```python
from build123d import *

# Parameters (mm, degrees)
SKETCH1_W           = 106.68
SKETCH1_H           = 38.1
BOSS_EXTRUDE1_DEPTH = 12.7
SKETCH2_R           = 3.2639
CUT_EXTRUDE1_DEPTH  = 22.225
CUT_EXTRUDE2_START  = -22.225
SKETCH3_R           = 3.2639
CUT_EXTRUDE2_DEPTH  = 22.225


with BuildPart() as part:
    # Sketch1 → Boss-Extrude1 (new body)
    with BuildSketch(Plane.XY):
        Rectangle(SKETCH1_W, SKETCH1_H)
    extrude(amount=BOSS_EXTRUDE1_DEPTH)

    # Sketch2 → Cut-Extrude1 (cut)
    with BuildSketch(Plane(origin=(53.34, 0, 0), x_dir=(0, 0, -1), z_dir=(1, 0, 0))):
        with Locations((-6.35, 10.16)):
            Circle(SKETCH2_R)
        with Locations(Location((-6.35, -10.16, 0), (0, 0, 180))):
            Circle(SKETCH2_R)
    extrude(amount=-CUT_EXTRUDE1_DEPTH, mode=Mode.SUBTRACT)

    # Sketch3 → Cut-Extrude2 (cut)
    with BuildSketch(Plane.ZY.offset(53.34).offset(CUT_EXTRUDE2_START)):
        with Locations(Location((6.35, 10.16, 0), (0, 0, 180))):
            Circle(SKETCH3_R)
        with Locations((6.35, -10.16)):
            Circle(SKETCH3_R)
    extrude(amount=CUT_EXTRUDE2_DEPTH, mode=Mode.SUBTRACT)


solid = part.part
```
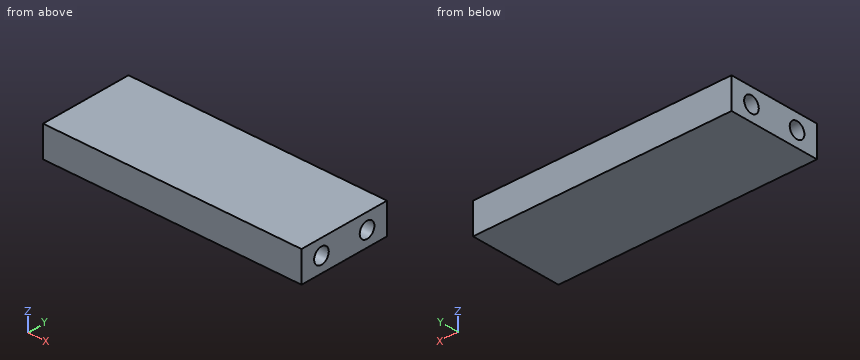
Could you check a few things on this model? Use its own coordinates, in mm. Coordinates: 2 decimals unless noted, no trailing zeros. Write each loop counter-clockwise with the first axis right and the second up, starting at its lowest first coordinate (ties: lowest second). Pieces come first, ordered by that corner, then holes. Notation, with made-up numbers: (-17, 36) -> (38, 36) arc R21 cw to (38, 75) -> close; hole circle Ø6 at (-22.75, 48). An arc over 180 degrees is marked (long way). Return JSON: item names as keys, results as strings.
(1) I need wall thicknesses on L1, parallel to Y at x = 39.25, z = 6.35; L2, parallel to X at y = 10, z = 7.5 (3 decimals); L3, parallel to Z at x = -44.5, y = 10.16. Which ranges of each line are inside material? Lowest first, please.
Numbers:
{"L1": "y = -19.05 to -13.42, -6.9 to 6.9, 13.42 to 19.05", "L2": "x = -31.115 to 31.115", "L3": "z = 0 to 3.09, 9.61 to 12.7"}
(2) I'm going to push flat-ended pins straight in: pin 1 (4 mm diameter, centred on y = -10.16, z = 6.35, fed in from -X) (3 decimals); pin 2 (2 mm diameter, centred on y = 11, z = 6, fed in from +X) (3 decimals). Where does each tip first touch, or does it pass through?
Numbers:
{"pin 1": "stops at x = -31.115", "pin 2": "stops at x = 31.115"}
(3) Imagine slicing it at B-B, the plane z = 7.5. Please give me the cut outline in (x, y) (3 decimals), then the cut area to 3 significant figures.
Numbers:
{"outline": "(-53.34, -19.05) -> (53.34, -19.05) -> (53.34, -13.215) -> (31.115, -13.215) -> (31.115, -7.105) -> (53.34, -7.105) -> (53.34, 7.105) -> (31.115, 7.105) -> (31.115, 13.215) -> (53.34, 13.215) -> (53.34, 19.05) -> (-53.34, 19.05) -> (-53.34, 13.215) -> (-31.115, 13.215) -> (-31.115, 7.105) -> (-53.34, 7.105) -> (-53.34, -7.105) -> (-31.115, -7.105) -> (-31.115, -13.215) -> (-53.34, -13.215) -> close", "area": "3,520 mm2"}
(4) Imagine slicing it at A-A, the plane y = -10.16. Please give me the cut outline in (x, z) (3 decimals), then the cut area to 3 significant figures.
Numbers:
{"outline": "(-53.34, 0) -> (53.34, 0) -> (53.34, 3.086) -> (31.115, 3.086) -> (31.115, 9.614) -> (53.34, 9.614) -> (53.34, 12.7) -> (-53.34, 12.7) -> (-53.34, 9.614) -> (-31.115, 9.614) -> (-31.115, 3.086) -> (-53.34, 3.086) -> close", "area": "1,060 mm2"}
